Could you check a few things on this drawing? It's one solid part, dimensions in mm from its lowest x, y, z. A direction names the side the tool comes from. Coordinates: 2 decimals unless noted, no trailing zeros. Order: outer loops, then holes, each group sorted by start corner. A loop starts at its lowest first (then second) coordinate and runs counter-clockwise, first axis right, second up. Notation, with made-up numbers: (73, 32.5) -> (112, 32.5) arc R13 cw to (112, 46.5) -> close; hole circle Ø7 at (87, 80). An arc over 180 degrees is marked (long way). Answer as CSV lines item,"result".
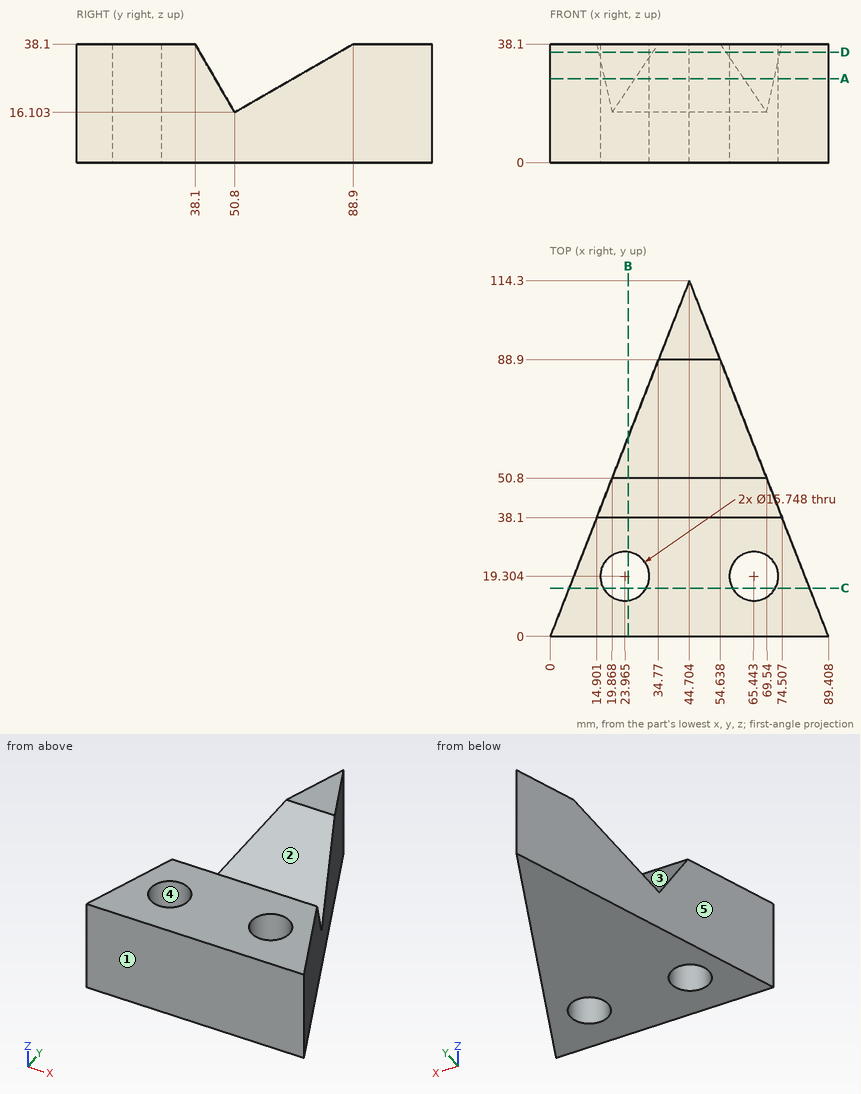
Q1. We'd pull the mould along X, two halves only. Please class the marked faces 3, 4 and 5: pulls with the +X half, pulls with the -X half, needs draft (parallel to the pull), parting line crosses it, or undercut.
Solution:
face 3,"needs draft"
face 4,"undercut"
face 5,"pulls with the -X half"
Q2. If I drill on line 1 (X direction, y = 22, z = 31) (1 decimal); line 2 (X direction, y = 23.5, z = 17.5) (1 decimal); line 3 (Y direction, x = 66.5, z = 30.5) (1 decimal), over which ranges is the centre line in solid material (lowest first)?
Solution:
line 1,"8.6 to 16.6, 31.4 to 58, 72.8 to 80.8"
line 2,"9.2 to 17.3, 30.6 to 58.8, 72.1 to 80.2"
line 3,"0 to 11.5, 27.1 to 42.5"
Q3. For P1, Ø1.5, axis at y = 89.5, z = 8.5, coming from the -X side; P2, Ø12.5, axis at x = 23.97, y = 19.3, coming from the -Z side; P3, Ø4, axis at y = 63, z = 19.5, coming from the -X side; P4, Ø1.5, axis at y = 26.5, z = 25, coming from the +X side, each with a flat end and sliding along its axis, tell me the tip position at first contact or that it passes through.
Solution:
P1,"x = 34.71"
P2,"through"
P3,"x = 23.86"
P4,"x = 79.34"
Q4. Imagine slicing it at D-D (z = 35.5). List the corners of the cut face in (x, y) for me (1 decimal), and give its area (3 significant figures).
Solution:
outline,"(0, 0) -> (89.4, 0) -> (73.9, 39.6) -> (15.5, 39.6) -> close; (33, 84.4) -> (56.4, 84.4) -> (44.7, 114.3) -> close; hole circle Ø15.7 at (24, 19.3); hole circle Ø15.7 at (65.4, 19.3)"
area,"2,890 mm2"
Q5. Imagine slicing it at B-B (x = 25). List the corners of the cut face in (y, z) for me.
Solution:
outline,"(0, 0) -> (11.5, 0) -> (11.5, 38.1) -> (0, 38.1) -> close; (27.11, 0) -> (63.92, 0) -> (63.92, 23.68) -> (50.8, 16.1) -> (38.1, 38.1) -> (27.11, 38.1) -> close"
Q6. Imagine slicing it at C-C (y = 15.5). List the corners of the cut face in (x, z) for me (1 decimal), and give its area (3 significant figures).
Solution:
outline,"(6.1, 0) -> (17.1, 0) -> (17.1, 38.1) -> (6.1, 38.1) -> close; (30.9, 0) -> (58.5, 0) -> (58.5, 38.1) -> (30.9, 38.1) -> close; (72.3, 0) -> (83.3, 0) -> (83.3, 38.1) -> (72.3, 38.1) -> close"
area,"1,890 mm2"
Q7. Which directions (+Z, -Z, +X, -X, +Y, -Y) give clear straight access to the entire face, cutting with the end or side of a thin tool? Please do the marked faces 1 and 2.
Solution:
face 1,"+Z, -Z, +X, -X, -Y"
face 2,"+Z, +X, -X"
Q8. Imagine slicing it at A-A (z = 27). Give the number of separate pieces and of enclosed holes in the cut face, and give its area (3 significant figures).
Solution:
separate pieces,"2"
enclosed holes,"2"
area,"3,590 mm2"
